Design review of the part built by this model. Coordinates are the model's own, in mm. A direction names the side the tool comes from. Coordinates: 2 decimals unless noted, no trailing zeros. Use a Markdown table: item, result. Add a question column.
Q1. Draft analysis for pull direction Y (two halves, no side actions). For faces 1 (the face through (-3.525, -5.952, 1.565)), 2 (the face through (-4.932, 4.827, 1.565)), 3 (the face through (-6.65, -1.86, 1.57)), state which applies: pulls with the +Y half, pulls with the -Y half, needs draft (parallel to the pull), parting line crosses it, or undercut.
Q2. For probe 1 along X at (y, z) = (-1.25, 0.75); probe 2 along X at (y, z) = (-0.75, 0.65); probe 3 along Y at (x, z) = (5.75, 1.15), list the stretches that pass through material, from the lowest coordinate up.
Q3. For faces 4 (the face through (-4.827, -4.932, 1.565)), 5 (the face through (-3.849, 5.035, 1.565)), 6 (the face through (6.917, -0.076, 1.565)), 7 (the face through (-0.816, 6.285, 1.565)), list the 3-axis set-ups (+Z, -Z, +X, -X, +Y, -Y) from which the entire face can be reached by the end or side of a thin tool; tool diameter is ignored.
from build123d import *

# Parameters (mm, degrees)
F0_R     = 1.905
F1_DEPTH = 3.175
F2_COUNT = 12


# Not quite as in the source:
# - a length typed as a fraction of an inch, garbled in the dataset ("3 / 203.2 mm" for 3/8 in), is restored


with BuildPart() as f1:
    # F0 (on Top) → F1 (new body)
    with BuildSketch(Plane.XY):
        with BuildLine():
            ThreePointArc((0, 6.3373), (-4.4811478044, -4.4811478044), (6.3373, 0))
            ThreePointArc((6.3373, 0), (5.0277181234, 3.8579038041), (1.6402139345, 6.1213617389))
            ThreePointArc((1.6402139345, 6.1213617389), (0.827183638, 6.28308352), (0, 6.3373))
        make_face()
        Circle(F0_R, mode=Mode.SUBTRACT)
        with BuildLine():
            ThreePointArc((0, 6.3373), (0.827183638, 6.28308352), (1.6402139345, 6.1213617389))
            Line((1.6402139345, 6.1213617389), (1.7907858552, 7.2650690248))
            ThreePointArc((1.7907858552, 7.2650690248), (1.7153129857, 7.5467376085), (1.4627758423, 7.6925399962))
            Line((1.4627758423, 7.6925399962), (0.5780428921, 7.8090172988))
            ThreePointArc((0.5780428921, 7.8090172988), (0.2963743084, 7.7335444293), (0.1505719207, 7.4810072858))
            Line((0.1505719207, 7.4810072858), (0, 6.3373))
        make_face()
    extrude(amount=F1_DEPTH)

    # F2: F1 ×12 about axis
    f2_axis = Axis((0, 0, 0), (0, 0, -1))


with BuildPart() as f1_1:
    add(f1.part)
    for i in range(1, F2_COUNT):
        add(f1.part.rotate(f2_axis, i * 360 / F2_COUNT))


solid = f1_1.part
Answer list:
| question | item | result |
|---|---|---|
| 1 | face 1 | pulls with the -Y half |
| 1 | face 2 | pulls with the +Y half |
| 1 | face 3 | undercut |
| 2 | probe 1 | -6.21 to -1.44, 1.44 to 7.72 |
| 2 | probe 2 | -6.29 to -1.75, 1.75 to 7.79 |
| 2 | probe 3 | -5.24 to -3.37, -2.66 to 3.28 |
| 3 | face 4 | +Z, -Z, -X |
| 3 | face 5 | +Z, -Z |
| 3 | face 6 | +Z, -Z, +X |
| 3 | face 7 | +Z, -Z, +Y |
